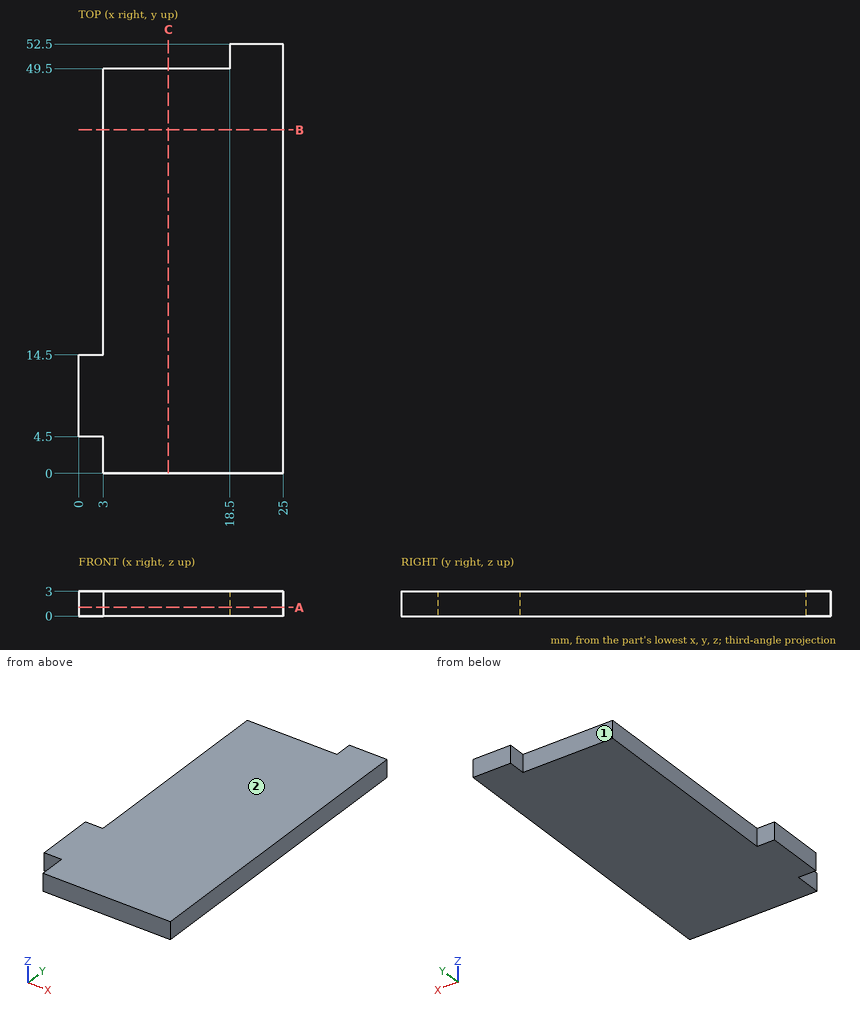
Geometry: see drawing. Coordinates: mm, zero at the bounding-box minimum. A direction names the side the tool comes from. Round coordinates to 2 decimals unless told otherwise and drop trailing zeros. Loops run counter-clockwise (first coordinate to the right, second up) from the corner with the lowest first, then second, coordinate; pieces in that order, holes last. Notation, with made-up numbers: (60, -27) -> (70, -27) arc R8 cw to (70, -23) -> close; hole circle Ø10 at (-3.5, 78.5). An arc over 180 degrees is marked (long way). One line per question, with ' | ' between items. Start each with the question number.
1. Section B-B on y = 42. Output: boundary loops of the cut face in (x, z).
2. Section A-A on z = 1.05. Output: boundary loops of the cut face in (x, y), and give its area (3 significant figures).
3. Section C-C on x = 11. Output: boundary loops of the cut face in (y, z), and give its area (4 significant figures).
4. Contact query for flat-ended pins moving along their axis: pin 1 (1 mm diameter, centred on x = 14.5, z = 1.5, fed in from +Y); pin 2 (2 mm diameter, centred on x = 12.5, y = 14.5, fed in from -Z). Output: stop coordinate, or through.
5. Set-up query: the marked faces 1 and 2. Return all of +Z, -Z, +X, -X, +Y, -Y with unobstructed straight access to the full face (end or side cutting, diameter ignored); none if empty.
6. Line query: line 1 along X through (y, z) = (44, 2.9); line 2 along Y through (x, z) = (13.25, 2.3); line 3 along Y through (x, z) = (2.25, 1.15). Output: solid intervals per line, ascending. Write a range as [from, to].
Returned:
1) outline: (3, 0) -> (25, 0) -> (25, 3) -> (3, 3) -> close
2) outline: (0, 4.5) -> (3, 4.5) -> (3, 0) -> (25, 0) -> (25, 52.5) -> (18.5, 52.5) -> (18.5, 49.5) -> (3, 49.5) -> (3, 14.5) -> (0, 14.5) -> close | area: 1,140 mm2
3) outline: (0, 0) -> (49.5, 0) -> (49.5, 3) -> (0, 3) -> close | area: 148.5 mm2
4) pin 1: stops at y = 49.5 | pin 2: stops at z = 0
5) face 1: +Z, -Z, -X, +Y | face 2: +Z, +X, -X, +Y, -Y
6) line 1: x = [3, 25] | line 2: y = [0, 49.5] | line 3: y = [4.5, 14.5]
